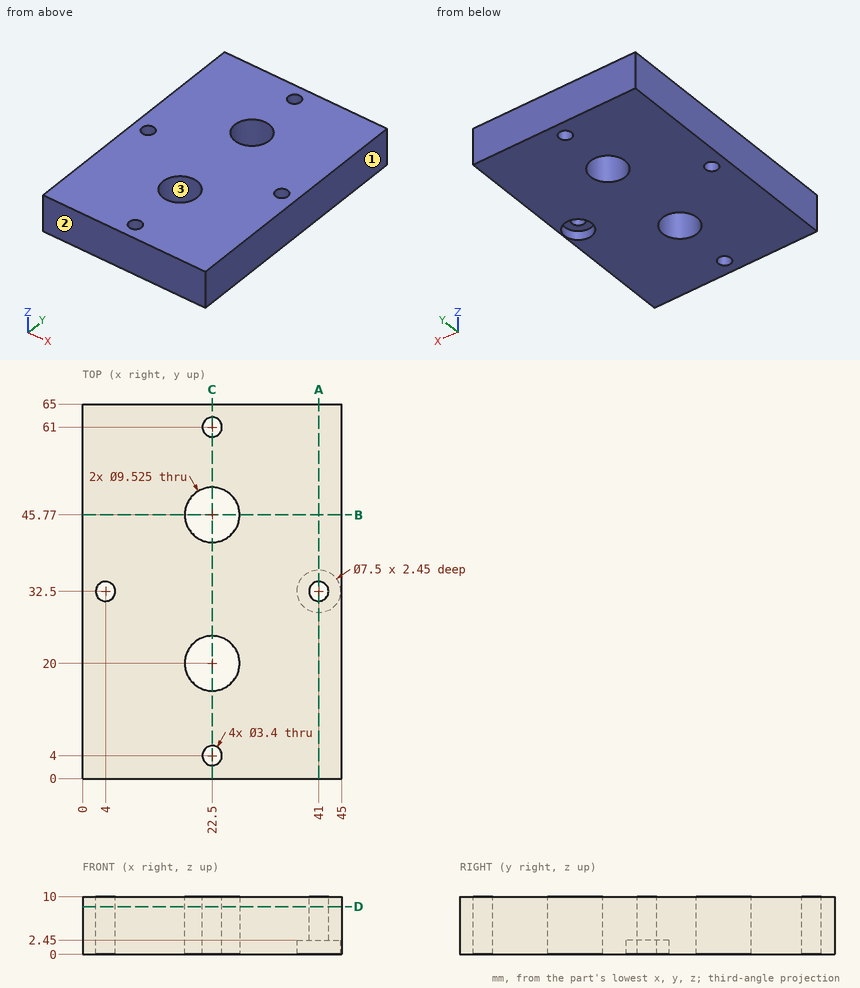
The drawing under review shows one solid part. Ordinate dimensions are in mm from its lowest x, y, z. Round coordinates to 2 decimals unless told otherwise and drop trailing zeros. Loops run counter-clockwise (first coordinate to the right, second up) from the corner with the lowest first, then second, coordinate; pieces in that order, holes last. Notation, with made-up numbers: (-18.5, 47.5) - (15.5, 47.5) arc R25 cw to (15.5, 81.5) - close; hole circle Ø3 at (53, 47.25). An arc over 180 degrees is marked (long way). One line per item, written item: value. Start each with the question number.
1) Insertion check: pin 1 Ø4.5 at (x, y) = (41, 32.5) entering from -Z. The pin has a flat end and moves straight along its axis. Give the tip position at first contact, or say it passes through.
2) Consider section D-D on z = 8.25. Give the boundary of the cut face in (x, y) (1 decimal), then the cut area to 3 significant figures.
3) To check wall thickness, follow L1, parallel to Y at x = 22.5, z = 6; L2, parallel to Y at x = 23, z = 2.5; L3, parallel to X at y = 61, z = 2. State the ranges of each line that lie inside material, in increasing order. Write a range as from..to.
4) Draft analysis for pull direction X (two halves, no side actions). For the marked faces 1, 2 and 3, state which applies: +X half, -X half, draft (parallel to the pull), parting line (faces both ways), or undercut.
5) Consider section B-B on y = 45.77. Give the boundary of the cut face in (x, z), then the cut area to 3 significant figures.
6) Consider section A-A on x = 41. Give the boundary of the cut face in (y, z).
7) Consider section C-C on x = 22.5. Give the boundary of the cut face in (y, z).
Reported:
1. pin 1: stops at z = 2.45
2. outline: (0, 0) - (45, 0) - (45, 65) - (0, 65) - close; hole circle Ø3.4 at (4, 32.5); hole circle Ø9.5 at (22.5, 20); hole circle Ø9.5 at (22.5, 45.8); hole circle Ø3.4 at (22.5, 4); hole circle Ø3.4 at (22.5, 61); hole circle Ø3.4 at (41, 32.5)
2. area: 2,750 mm^2
3. L1: y = 0..2.3, 5.7..15.24, 24.76..41.01, 50.53..59.3, 62.7..65
3. L2: y = 0..2.38, 5.62..15.26, 24.74..41.03, 50.51..59.38, 62.62..65
3. L3: x = 0..20.8, 24.2..45
4. face 1: +X half
4. face 2: draft
4. face 3: undercut
5. outline: (0, 0) - (17.74, 0) - (17.74, 10) - (0, 10) - close; (27.26, 0) - (45, 0) - (45, 10) - (27.26, 10) - close
5. area: 355 mm^2
6. outline: (0, 0) - (28.75, 0) - (28.75, 2.45) - (30.8, 2.45) - (30.8, 10) - (0, 10) - close; (34.2, 2.45) - (36.25, 2.45) - (36.25, 0) - (65, 0) - (65, 10) - (34.2, 10) - close
7. outline: (0, 0) - (2.3, 0) - (2.3, 10) - (0, 10) - close; (5.7, 0) - (15.24, 0) - (15.24, 10) - (5.7, 10) - close; (24.76, 0) - (41.01, 0) - (41.01, 10) - (24.76, 10) - close; (50.53, 0) - (59.3, 0) - (59.3, 10) - (50.53, 10) - close; (62.7, 0) - (65, 0) - (65, 10) - (62.7, 10) - close
